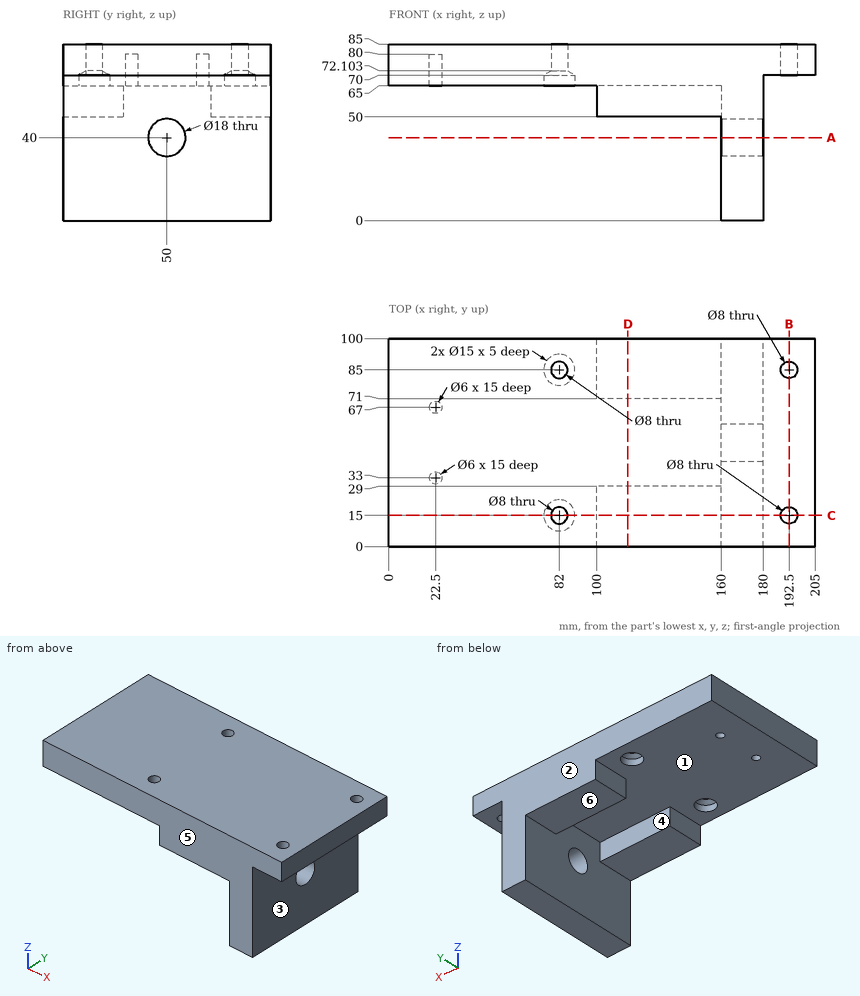
Check sheet for the drawn part. Datum: minimum x, y, z corner. Units: mm. A direction names the side the tool comes from. Give positions to 0.01 mm unless a question says otherwise; leave off trailing zeros. Loops run counter-clockwise (first coordinate to the right, second up) from the corner with the lowest first, then second, coordinate; pieces in that order, holes last.
1) Thickness scan on line 1 along Y through (x, z) = (82, 78); line 2 along Y through (x, z) = (82, 66); line 3 along X through (y, z) = (59, 69). Record the ranges inside material, lowest first.
2) Depth check by flat-ended pin: pin 1 Ø3 at (x, y) = (21.5, 66) entering from -Z; pin 2 Ø5 at (x, y) = (93.5, 24.5) entering from -Z; pin 3 Ø14.5 at (x, y) = (124, 84) entering from -Z; pin 4 Ø14.5 at (y, z) = (50, 40) entering from -X. Enter the tip coordinate at first touch or a pass-through.
3) Sectioned sample at A-A, the plane z = 40. Enter the section's corners in (x, y).
4) Sectioned sample at B-B, the plane x = 192.5. Enter the section's corners in (y, z).
5) Sectioned sample at C-C, the plane y = 15. Enter the section's corners in (x, z).
6) Draft check along Y on the marked faces 1, 2 and 3. Enter one of: pulls with the +Y half, pulls with the -Y half, needs draft (parallel to the pull), parting line crosses it, or undercut.
7) Set-up check for the marked faces 4, 5 and 6: record each of +Z, -Z, +X, -X, +Y, -Y from which the full face is reachable in a straight line by a thin tool's end or side.
8) Sectioned sample at D-D, the plane x = 115. Enter the section's corners in (y, z), then the cut area to 3 significant figures.
Answers:
1. line 1: y = 0 to 11, 19 to 81, 89 to 100
1. line 2: y = 0 to 7.5, 22.5 to 77.5, 92.5 to 100
1. line 3: x = 0 to 180
2. pin 1: stops at z = 80
2. pin 2: stops at z = 65
2. pin 3: stops at z = 50
2. pin 4: passes through
3. outline: (160, 0) - (180, 0) - (180, 41) - (160, 41) - close; (160, 59) - (180, 59) - (180, 100) - (160, 100) - close
4. outline: (0, 70) - (11, 70) - (11, 85) - (0, 85) - close; (19, 70) - (81, 70) - (81, 85) - (19, 85) - close; (89, 70) - (100, 70) - (100, 85) - (89, 85) - close
5. outline: (0, 65) - (74.5, 65) - (74.5, 70) - (78, 72.1) - (78, 85) - (0, 85) - close; (86, 72.1) - (89.5, 70) - (89.5, 65) - (100, 65) - (100, 50) - (160, 50) - (160, 0) - (180, 0) - (180, 70) - (188.5, 70) - (188.5, 85) - (86, 85) - close; (196.5, 70) - (205, 70) - (205, 85) - (196.5, 85) - close
6. face 1: undercut
6. face 2: pulls with the +Y half
6. face 3: needs draft
7. face 4: -Z, -X
7. face 5: +Z, -Z, +X, -X, -Y
7. face 6: -Z, -X, +Y, -Y
8. outline: (0, 50) - (29, 50) - (29, 65) - (71, 65) - (71, 50) - (100, 50) - (100, 85) - (0, 85) - close
8. area: 2,870 mm2
